Geometry: final body of the model. Coordinates: model frame, mm. A direction names the side the tool comes from. Coordinates: 2 decimals unless noted, no trailing zeros. Loops run counter-clockwise (first coordinate to the right, second up) from the corner with the lowest first, then second, coordinate; pieces in that order, holes last. Notation, with made-up numbers: (65, 19.25) - (87, 19.25) arc R19 ccw to (87, 49.25) - close; hole circle Ø4 at (24.25, 6.5). An arc over 180 degrees is marked (long way). Answer in a Markdown table with one row per item.
Autodesk Fusion 360 part; units mm, degrees
sketch "Front" plane through (0, 0, 0) normal (0, 1, 0) x (1, 0, 0)
  line L0 (-15, -25) -> (15, -25)
  line L1 (15, -25) -> (15, 25)
  line L2 (15, 25) -> (-15, 25)
  line L3 (-15, 25) -> (-15, -25)
  line L4 (0, -25) -> (0, 25) construction
  circle A0 centre (0, 10) radius 4
  circle A1 centre (0, -10) radius 3.5
  circle A2 centre (0, 10) radius 7.5
  dimension "d11" = 30
  dimension "d12" = 50
  dimension "d19" = 8
  dimension "d20" = 7
  dimension "d21" = 20
  dimension "d24" = 15
  dimension "d26" = 15
extrude "Extrude3" add sketch "Front" against normal blind 10 contours A2
extrude "Extrude4" add sketch "Front" against normal blind 18 contours L0 L1 L2 L3
(1) Pull-direction query (Z, two-part tool) for faces 3 (the face through (3, -10, -7)), 4 (the face through (0, -9, 25)), 5 (the face through (-15, -9, 0)), 6 (the face through (-0.759, -8.874, 13.417)); classes: pulls with the +Z half, pulls with the -Z half, needs draft (parallel to the pull), parting line crosses it, or undercut.
Verdict:
| item | result |
|---|---|
| face 3 | undercut |
| face 4 | pulls with the +Z half |
| face 5 | needs draft |
| face 6 | undercut |
(2) Cut plane D-D on z = -10. Output: boundary loops of the cut face in (x, y).
Verdict:
| item | result |
|---|---|
| outline | (-15, -18) - (-7.5, -18) - (-7.5, -10) - (-4, -10) - (-4, 0) - (-15, 0) - close; (4, -10) - (7.5, -10) - (7.5, -18) - (15, -18) - (15, 0) - (4, 0) - close |
(3) Access query for faces 1 (the face through (-1.63, -13.94, -2.68)), 2 (the face through (15, -9, 0)). Directions: +Z, -Z, +X, -X, +Y, -Y. A direction counts if a zero-diameter tool reaches every point of the face in a straight line with its end or side. Return the directions, or none.
Verdict:
| item | result |
|---|---|
| face 1 | -Y |
| face 2 | +Z, -Z, +X, +Y, -Y |
(4) Ray query, probe 1 along Z at (x, y) = (0, -13.25); probe 2 along X at (y, z) = (-4.75, 10); probe 3 along X at (y, z) = (-14, -10). Return the intervals inside material, ascending.
Verdict:
| item | result |
|---|---|
| probe 1 | z = -25 to -17.5, -2.5 to 6.5, 13.5 to 25 |
| probe 2 | x = -15 to -3.5, 3.5 to 15 |
| probe 3 | x = -15 to -7.5, 7.5 to 15 |
(5) Cut plane A-A on x = 0. Output: boundary loops of the cut face in (y, z), then the cut area to 3 significant figures.
Verdict:
| item | result |
|---|---|
| outline | (-18, -25) - (0, -25) - (0, -14) - (-10, -14) - (-10, -17.5) - (-18, -17.5) - close; (-18, -2.5) - (-10, -2.5) - (-10, -6) - (0, -6) - (0, 6.5) - (-18, 6.5) - close; (-18, 13.5) - (0, 13.5) - (0, 25) - (-18, 25) - close |
| area | 574 mm² |
(6) Cut plane B-B on z = 10. Output: boundary loops of the cut face in (x, y), then the cut area to 3 significant figures.
Verdict:
| item | result |
|---|---|
| outline | (-15, -18) - (-3.5, -18) - (-3.5, 0) - (-15, 0) - close; (3.5, -18) - (15, -18) - (15, 0) - (3.5, 0) - close |
| area | 414 mm² |
(7) Cut plane C-C on y = -13.5. Output: boundary loops of the cut face in (x, z).
Verdict:
| item | result |
|---|---|
| outline | (-15, -25) - (15, -25) - (15, 25) - (-15, 25) - close; hole circle Ø15 at (0, -10); hole circle Ø7 at (0, 10) |
